Work out the finished part from the listing and answer in its coordinate system (mm). Give positions to 0.01 mm unless a question says otherwise; leave off trailing zeros. Order: outer loops, then holes, each group sorted by start corner. A loop starts at its lowest first (then second) coordinate and runs counter-clockwise, first axis right, second up.
```python
from build123d import *

# Parameters (mm, degrees)
F0_W     = 158.75
F0_H     = 65.0748
F0_R     = 5.3975
F1_DEPTH = 3.175


with BuildPart() as f1:
    # F0 (on Top) → F1 (new body)
    with BuildSketch(Plane.XY):
        with Locations((79.375, 32.5374)):
            Rectangle(F0_W, F0_H)
        with Locations((15.0876, 14.2875)):
            Circle(F0_R, mode=Mode.SUBTRACT)
        with Locations((143.6624, 14.2875)):
            Circle(F0_R, mode=Mode.SUBTRACT)
        Polygon((0, 103.4796), (0, 65.0748), (158.75, 65.0748), (158.75, 85.6996), align=None)
    extrude(amount=F1_DEPTH)


solid = f1.part
```
1. The part is cut by section A-A (z = 0.9). State how many separate pieces and enclosed holes the cut face has, then the cut area to 3 significant figures.
Findings below:
separate pieces: 1
enclosed holes: 2
area: 14,800 mm2
2. The part is cut by section B-B (x = 33). Write down the section's boundary in (y, z) (3 decimals), then the cut area to 3 significant figures.
Findings below:
outline: (0, 0) - (99.784, 0) - (99.784, 3.175) - (0, 3.175) - close
area: 317 mm2
3. The mould has two halves that part along Y. Classify faces 1 (the face through (17.58, 9.5, 1.57)), 2 (the face through (80.486, 94.465, 1.565)), 3 (the face through (158.75, 42, 2)), 4 (the face through (148.81, 15.91, 1.57)): pulls with the +Y half, pulls with the -Y half, needs draft (parallel to the pull), parting line crosses it, or undercut.
Findings below:
face 1: undercut
face 2: pulls with the +Y half
face 3: needs draft
face 4: undercut
4. Straight lines are drawn through the part: probe 1 along X at (y, z) = (13, 2.4); probe 2 along Y at (x, z) = (143.5, 2.6); probe 3 along Y at (x, z) = (10.5, 0.4). For each, find the intervals that lie inside material, in ascending order.
Findings below:
probe 1: x = 0 to 9.85, 20.33 to 138.42, 148.9 to 158.75
probe 2: y = 0 to 8.89, 19.68 to 87.41
probe 3: y = 0 to 11.44, 17.13 to 102.3
5. The part is cut by section C-C (x = 93). Write down the section's boundary in (y, z) (3 decimals), then the cut area to 3 significant figures.
Findings below:
outline: (0, 0) - (93.064, 0) - (93.064, 3.175) - (0, 3.175) - close
area: 295 mm2
6. Given P1, Ø1.5, axis at x = 24, y = 66.5, coming from the -Z side, flat-ended and moving along its own axis, determine where the tip first touches the part or whether it passes through.
Findings below:
P1: stops at z = 0
